Print and shaded views of the part. All mm, measured from the part's lowest x, y and z. A direction names the side the tool comes from. Round coordinates to 2 decimals unless told otherwise and drop trailing zeros. Loops run counter-clockwise (first coordinate to the right, second up) from the corner with the lowest first, then second, coordinate; pieces in that order, holes last. Notation, with made-up numbers: (22, 47.25) - (61, 47.25) arc R25 ccw to (61, 61.25) - close; hole circle Ø11 at (11.5, 27). An arc over 180 degrees is marked (long way). Answer as a JSON object with one key per item and string values.
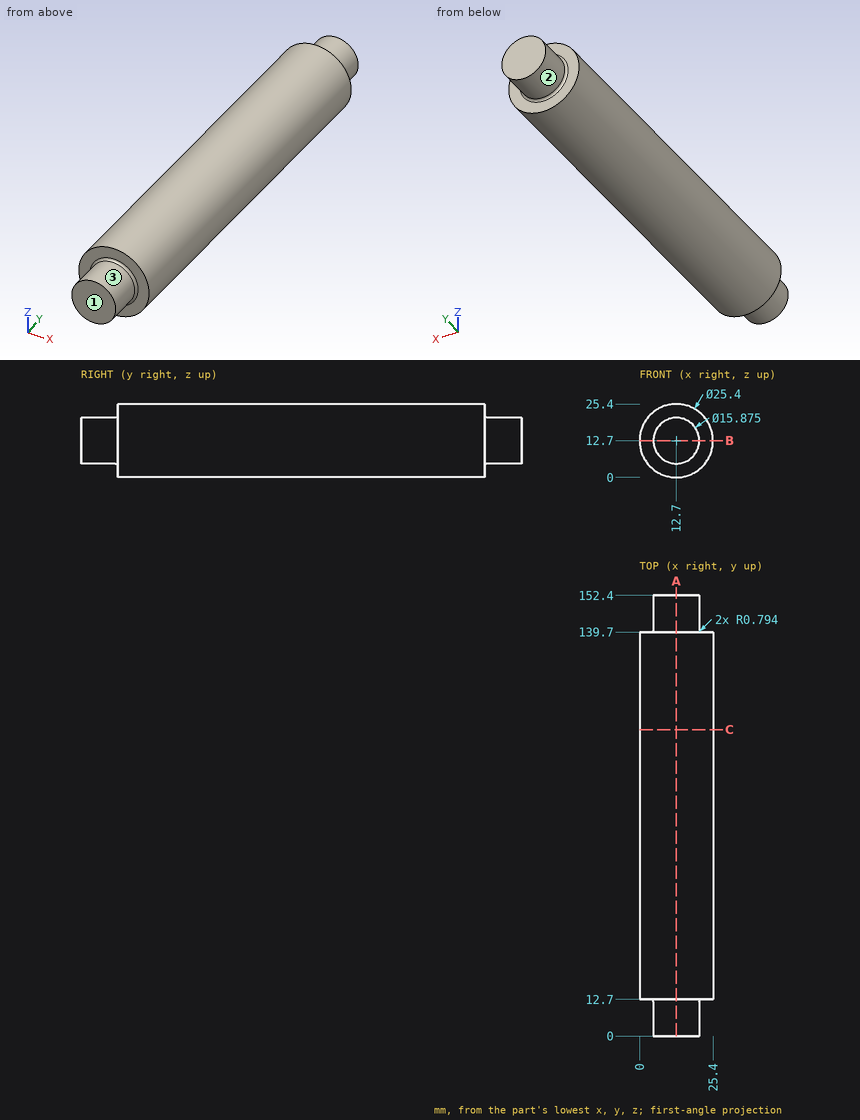
1) Tool access for the marked faces 1, 2 and 3: list every direction of +Z, -Z, +X, -X, +Y, -Y with a clear straight run to the whole face (end or side of a thin tool).
Values follow:
{"face 1": "+Z, -Z, +X, -X, -Y", "face 2": "+Y", "face 3": "-Y"}
2) Slice it at B-B on z = 12.7. List the corners of the cut face in (x, y), then the cut area to 3 significant figures.
Values follow:
{"outline": "(0, 12.7) - (3.97, 12.7) arc R0.79 cw to (4.76, 11.91) - (4.76, 0) - (20.64, 0) - (20.64, 11.91) arc R0.79 cw to (21.43, 12.7) - (25.4, 12.7) - (25.4, 139.7) - (21.43, 139.7) arc R0.79 cw to (20.64, 140.49) - (20.64, 152.4) - (4.76, 152.4) - (4.76, 140.49) arc R0.79 cw to (3.97, 139.7) - (0, 139.7) - close", "area": "3,630 mm²"}
3) Drop flat-ended pins along their axis: P1, Ø1.5, axis at y = 102.5, z = 14.5, coming from the +X side; P2, Ø1, axis at x = 19, z = 20, coming from the -Y side; P3, Ø1.5, axis at x = 8, y = 120, coming from the +Z side. Give the stop position or say it passes through.
Values follow:
{"P1": "x = 25.36", "P2": "y = 12.7", "P3": "z = 24.77"}
4) Probe probe 1 along Y at (x, z) = (16, 24.25); probe 2 along Z at (x, y) = (3.5, 62) (1 decimal); probe 3 along X at (y, z) = (121, 13.25). List the from-to ranges inside material, lowest first.
Values follow:
{"probe 1": "12.7 to 139.7", "probe 2": "3.9 to 21.5", "probe 3": "0.01 to 25.39"}
5) Slice it at A-A on x = 12.7. List the corners of the cut face in (y, z).
Values follow:
{"outline": "(0, 4.76) - (11.91, 4.76) arc R0.79 cw to (12.7, 3.97) - (12.7, 0) - (139.7, 0) - (139.7, 3.97) arc R0.79 cw to (140.49, 4.76) - (152.4, 4.76) - (152.4, 20.64) - (140.49, 20.64) arc R0.79 cw to (139.7, 21.43) - (139.7, 25.4) - (12.7, 25.4) - (12.7, 21.43) arc R0.79 cw to (11.91, 20.64) - (0, 20.64) - close"}
6) Slice it at C-C on y = 106. List the corners of the cut face in (x, z).
Values follow:
{"outline": "circle Ø25.4 at (12.7, 12.7)"}
